The figure shows three views and two pictorial views of one solid part (mm, origin at its lowest corner). Answer the questions. Coordinates: 2 decimals unless noted, no trailing zeros. Loops run counter-clockwise (first coordinate to the right, second up) from the corner with the lowest first, then second, coordinate; pieces in that order, holes last. Notation, with made-up numbers: M 36,65 L 42,65 A24 ccw 42,95 Z; hole C 71.5,-8.5 d4. An arc over 180 degrees is marked long. Answer as a JSON object with one key per item and string values. Group by question number.
1. A cutting plane is placed at B-B on z = 92. Give the vertices of the cut face in (x, y), and give its area (3 significant figures).
2. Given pin 1 (5 mm diameter, centred on x = 8, z = 92, fed in from +Y), flat-ended and moving along its own axis, determine where the tip first touches the part or whether it passes through.
3. A cutting plane is placed at A-A on x = 92. Give the vertices of the cut face in (y, z), and give its area (3 significant figures).
4. Straight lines are drawn through the part: L1, parallel to X at y = 2.4, z = 92; L2, parallel to Z at x = 50, y = 2.75; L3, parallel to X at y = 3.9, z = 8. For each, find the intervals that lie inside material, in ascending order.
5. A cutting plane is placed at C-C on z = 8. Give the vertices of the cut face in (x, y), and give its area (4 significant figures).
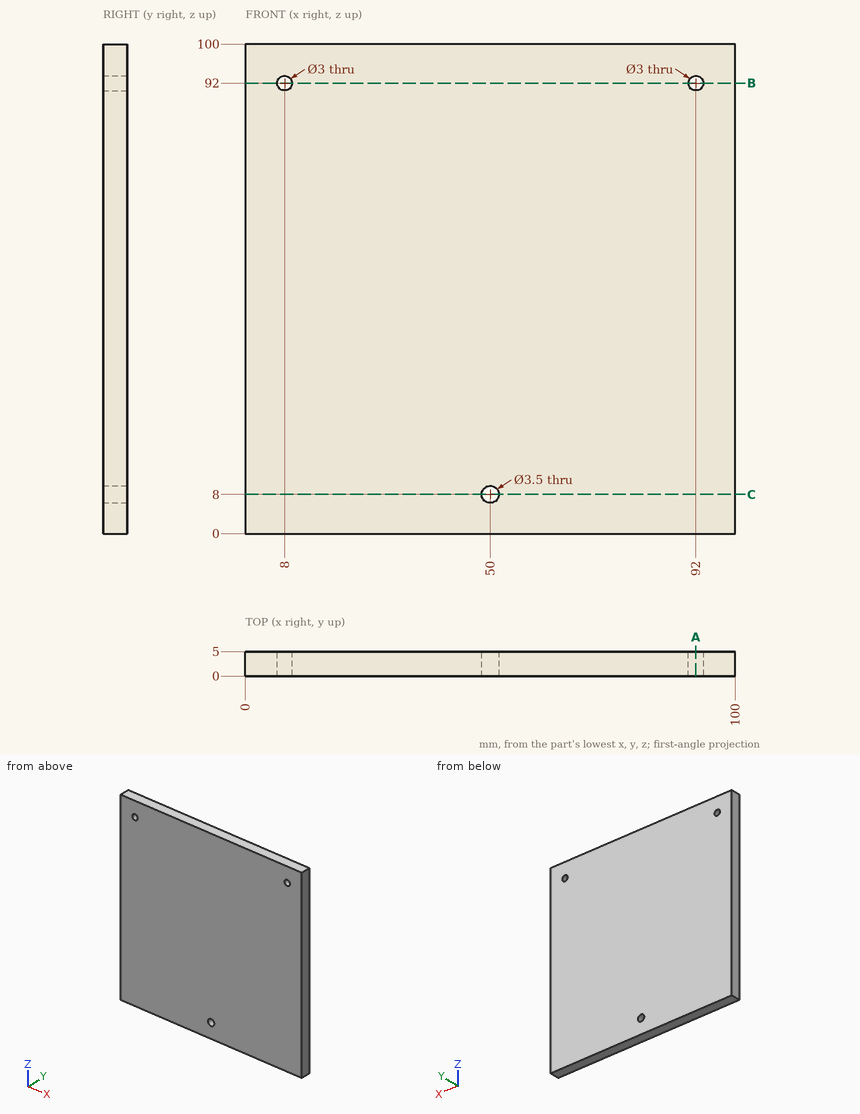
From the geometry:
{
 "1": {"outline": "M 0,0 L 6.5,0 L 6.5,5 L 0,5 Z; M 9.5,0 L 90.5,0 L 90.5,5 L 9.5,5 Z; M 93.5,0 L 100,0 L 100,5 L 93.5,5 Z", "area": "470 mm²"},
 "2": {"pin 1": "stops at y = 5"},
 "3": {"outline": "M 0,0 L 5,0 L 5,90.5 L 0,90.5 Z; M 0,93.5 L 5,93.5 L 5,100 L 0,100 Z", "area": "485 mm²"},
 "4": {"L1": "x = 0 to 6.5, 9.5 to 90.5, 93.5 to 100", "L2": "z = 0 to 6.25, 9.75 to 100", "L3": "x = 0 to 48.25, 51.75 to 100"},
 "5": {"outline": "M 0,0 L 48.25,0 L 48.25,5 L 0,5 Z; M 51.75,0 L 100,0 L 100,5 L 51.75,5 Z", "area": "482.5 mm²"}
}
